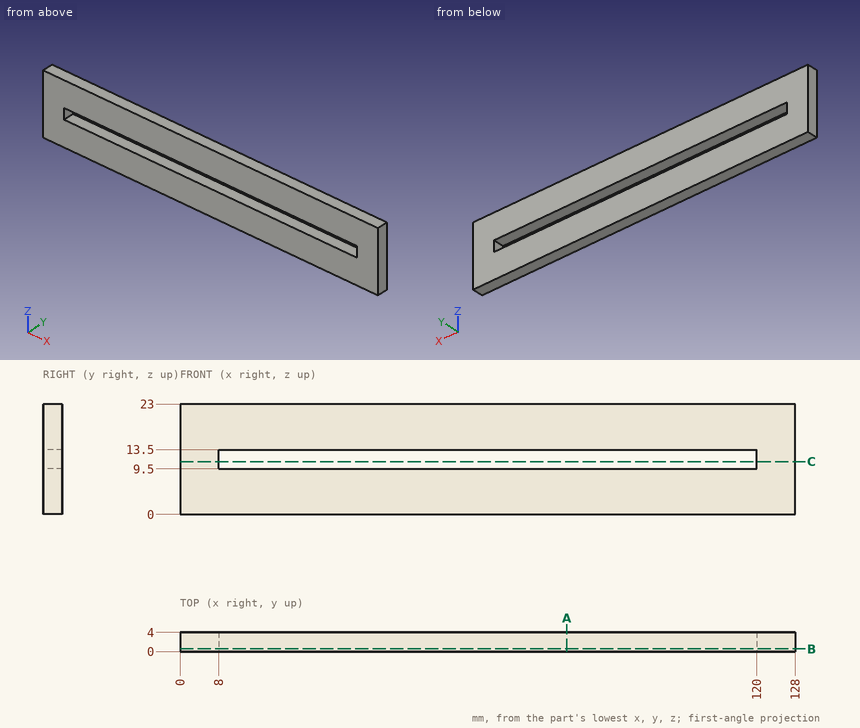
Geometry check sheet. Reference: drawing and pictorial views, mm from the part's lowest x, y, z. Round coordinates to 2 decimals unless told otherwise and drop trailing zeros. Loops run counter-clockwise (first coordinate to the right, second up) from the corner with the lowest first, then second, coordinate; pieces in that order, holes last. Notation, with made-up numbers: M 1,-11.5 L 26,-11.5 A24 cw 26,4.5 Z; hole C 33,-13.5 d6. An arc over 180 degrees is marked long. Return JSON: item names as keys, results as strings. Group by question number.
(1) Section check B-B, the plane y = 0.6. Enter the section's corners in (x, z), and give its area (3 significant figures).
(2) Section check C-C, the plane z = 11. Enter the section's corners in (x, y), and give its area (3 significant figures).
(3) Scan lines: line 1 along X through (y, z) = (3.2, 12.5); line 2 along Z through (x, y) = (71.5, 2.2). Record each from-to range of solid material in increasing order. Write a range as [from, to].
(4) Section check A-A, the plane x = 80.5. Enter the section's corners in (y, z).
Data:
{
 "1": {"outline": "M 0,0 L 128,0 L 128,23 L 0,23 Z; hole M 8,9.5 L 120,9.5 L 120,13.5 L 8,13.5 Z", "area": "2,500 mm²"},
 "2": {"outline": "M 0,0 L 8,0 L 8,4 L 0,4 Z; M 120,0 L 128,0 L 128,4 L 120,4 Z", "area": "64.0 mm²"},
 "3": {"line 1": "[0, 8], [120, 128]", "line 2": "[0, 9.5], [13.5, 23]"},
 "4": {"outline": "M 0,0 L 4,0 L 4,9.5 L 0,9.5 Z; M 0,13.5 L 4,13.5 L 4,23 L 0,23 Z"}
}
